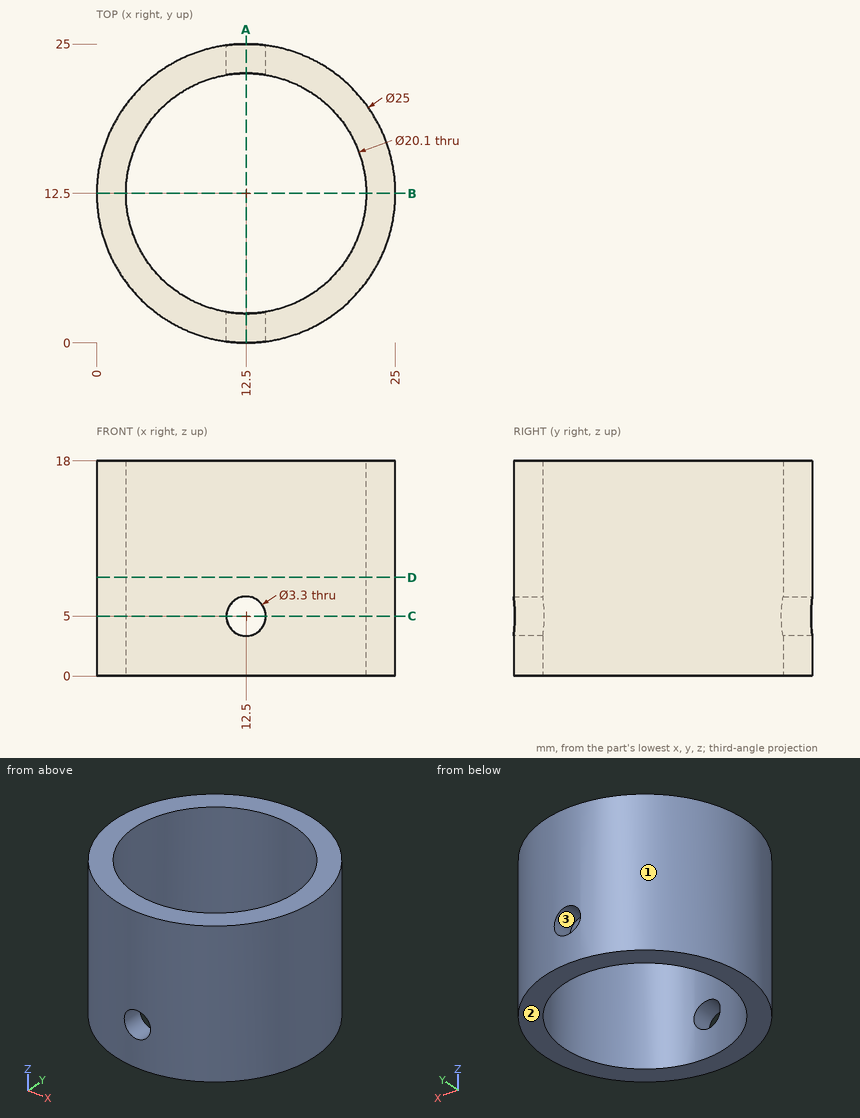
The figure shows three views and two pictorial views of one solid part (mm, origin at its lowest corner). Answer the questions. Round coordinates to 2 decimals unless told otherwise and drop trailing zeros. Loops run counter-clockwise (first coordinate to the right, second up) from the corner with the lowest first, then second, coordinate; pieces in that order, holes last. Notation, with made-up numbers: (-14, 25) -> (3, 25) arc R17 cw to (3, 38) -> close; hole circle Ø10 at (46, 20). An arc over 180 degrees is marked (long way). Use one line per item in the form item = value.
(1) Find section D-D on z = 8.25. Give the vertices of the cut face in (x, y), then the cut area to 3 significant figures.
Answer list:
outline = circle Ø25 at (12.5, 12.5); hole circle Ø20.1 at (12.5, 12.5)
area = 174 mm2
(2) Straight lines are drawn through the part: line 1 (Y direction, x = 12.75, z = 1.75); line 2 (Y direction, x = 5.75, z = 12.5). For each, find the intervals that lie inside material, in ascending order.
Answer list:
line_1 = 0 to 2.45, 22.55 to 25
line_2 = 1.98 to 5.05, 19.95 to 23.02
(3) Find section C-C on z = 5. Give the vertices of the cut face in (x, y).
Answer list:
outline = (10.85, 0.11) -> (10.85, 2.59) arc R10.05 cw to (10.85, 22.41) -> (10.85, 24.89) arc R12.5 ccw to start; (14.15, 0.11) arc R12.5 ccw to (14.15, 24.89) -> (14.15, 22.41) arc R10.05 cw to (14.15, 2.59) -> close
(4) Find section B-B on y = 12.5. Give the vertices of the cut face in (x, z), then the cut area to 3 significant figures.
Answer list:
outline = (0, 0) -> (2.45, 0) -> (2.45, 18) -> (0, 18) -> close; (22.55, 0) -> (25, 0) -> (25, 18) -> (22.55, 18) -> close
area = 88.2 mm2
(5) Find section A-A on x = 12.5. Give the vertices of the cut face in (y, z).
Answer list:
outline = (0, 0) -> (2.45, 0) -> (2.45, 3.35) -> (0, 3.35) -> close; (0, 6.65) -> (2.45, 6.65) -> (2.45, 18) -> (0, 18) -> close; (22.55, 0) -> (25, 0) -> (25, 3.35) -> (22.55, 3.35) -> close; (22.55, 6.65) -> (25, 6.65) -> (25, 18) -> (22.55, 18) -> close
(6) For a pull along X with two mould halves and no side action, classify the marked faces 1, 2 and 3 as released by +X, released by -X, zero draft, split by the parting line, or undercut.
Answer list:
face_1 = split by the parting line
face_2 = zero draft
face_3 = undercut
(7) Flat-ended cylindrical pins translate along their axes: P1, Ø5, axis at y = 8.5, z = 13.5, coming from the +X side; P2, Ø1, axis at y = 16.5, z = 11.5, coming from the -X side; P3, Ø1, axis at x = 21.5, y = 16.5, coming from the -Z side; P4, Ø2, axis at y = 3.5, z = 15.5, coming from the -X side. Find the tip coordinate at first contact, or state that the pin passes through.
Answer list:
P1 = 24.91
P2 = 0.5
P3 = 0
P4 = 2.9
